Check sheet for the drawn part. Datum: minimum x, y, z corner. Units: mm. Give positions to 0.01 mm unless a question says otherwise; leave off trailing zeros. Write each loop counter-clockwise with the first axis right and the second up, starting at its lowest first coordinate (ties: lowest second). Pieces come first, ordered by that corner, then holes. Notation, with made-up numbers: M 3,30 L 9,30 A7 cw 9,37 Z; hole C 56,87 d2. An arc over 180 degrees is marked long. Write item = value, one per line. Start each with the question number.
1) Sectioned sample at D-D, the plane y = 71. Record the cut outline in (x, z), then the cut area to 3 significant figures.
2) Sectioned sample at C-C, the plane z = 34. Record the cut outline in (x, y) (1 decimal), then the cut area to 3 significant figures.
3) Sectioned sample at A-A, the plane y = 12. Record the cut outline in (x, z), then the cut area to 3 significant figures.
4) Sectioned sample at B-B, the plane x = 10. Record the cut outline in (y, z), then the cut area to 3 significant figures.
5) Scan lines: L1, parallel to Z at x = 10, y = 18.5; L2, parallel to Z at x = 3.25, y = 99.5; L3, parallel to Y at x = 11.75, z = 31.5 (1 decimal). Record each from-to range of solid material in increasing order.
6) Gauge pin test, flat ends, axial feed: pin 1 (4 mm diameter, centred on x = 7, z = 25.5, fed in from +Y); pin 2 (8 mm diameter, centred on x = 12, z = 37.5, fed in from -Y). Record the tip position at first contact, or that the pin passes through.
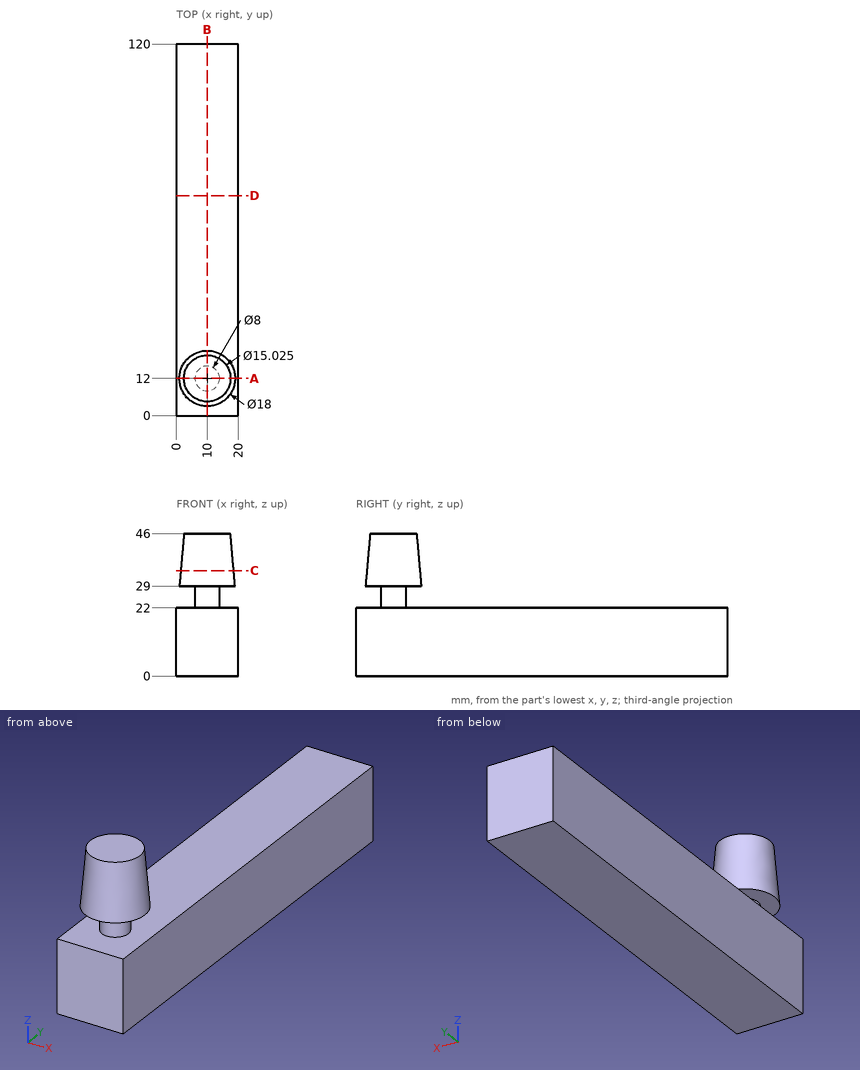
Data:
q1.outline = M 0,0 L 20,0 L 20,22 L 0,22 Z
q1.area = 440 mm2
q2.outline = C 10,12 d17.1
q2.area = 230 mm2
q3.outline = M 0,0 L 20,0 L 20,22 L 14,22 L 14,29 L 19,29 L 17.51,46 L 2.49,46 L 1,29 L 6,29 L 6,22 L 0,22 Z
q3.area = 777 mm2
q4.outline = M 0,0 L 120,0 L 120,22 L 16,22 L 16,29 L 21,29 L 19.51,46 L 4.49,46 L 3,29 L 8,29 L 8,22 L 0,22 Z
q4.area = 2,980 mm2
q5.L1 = 0 to 22, 29 to 46
q5.L2 = 0 to 22
q5.L3 = 3.4 to 20.6
q6.pin_1 = 15.87
q6.pin_2 = 3.43
